Work out the finished part from the listing and answer in its coordinate system (mm). A direction names the side the tool comes from. Round coordinates to 2 decimals unless told otherwise and drop trailing zeros. Write each loop counter-clockwise with the first axis right and the second up, starting at its lowest first coordinate (ties: lowest second). Pieces come first, ordered by that corner, then holes. Notation, with made-up numbers: (-35, 53.25) - (1, 53.25) arc R24 cw to (1, 88.25) - close; hole circle Ø1 at (46.25, 12). An arc over 180 degrees is marked (long way). Write item = value, one per line. Start each with the question number.
from build123d import *

# Parameters (mm, degrees)
PAD008_DEPTH    = 4.8
SKETCH012_W     = 5
SKETCH012_H     = 110
SKETCH012_H_2   = 105
SKETCH012_W_2   = 90
SKETCH012_H_3   = 5
PAD009_DEPTH    = 0.2
PAD010_DEPTH    = 6
SKETCH024_W     = 95
SKETCH024_H     = 120
PAD021_DEPTH    = 5.67
SKETCH025_W     = 65
SKETCH025_H     = 32.5
PAD022_DEPTH    = 2
FILLET004_R     = 3.5
SKETCH029_W     = 1.25
SKETCH029_H     = 105
POCKET006_DEPTH = 5
SKETCH030_W     = 70
SKETCH030_H     = 5
POCKET007_DEPTH = 15
FILLET006_R     = 4
SKETCH032_W     = 70
SKETCH032_H     = 7.5
POCKET008_DEPTH = 4


with BuildPart() as part:
    # Sketch011 → Pad008 (new body)
    with BuildSketch(Plane.XY):
        Polygon((0, 0), (95, 0), (95, -5), (95, -110), (86.25, -110), (86.25, -5), (8.75, -5), (8.75, -110), (0, -110), (0, -5), align=None)
    extrude(amount=PAD008_DEPTH)

    # Sketch012 (on Face12 of Pad008) → Pad009 (join)
    with BuildSketch(Plane.XY.offset(4.8)):
        with Locations((2.5, -55)):
            Rectangle(SKETCH012_W, SKETCH012_H)
        with Locations((92.5, -57.5)):
            Rectangle(SKETCH012_W, SKETCH012_H_2)
        with Locations((50, -2.5)):
            Rectangle(SKETCH012_W_2, SKETCH012_H_3)
    extrude(amount=PAD009_DEPTH)

    # Pad009 Face16 → Pad010 (add)
    with BuildSketch(Plane(origin=(47.5, -40.368852, 5), x_dir=(0, 1, 0), z_dir=(0, 0, 1))):
        Polygon((40.368852, 42.5), (40.368852, 47.5), (-69.631148, 47.5), (-69.631148, 42.5), (35.368852, 42.5), (35.368852, -42.5), (-69.631148, -42.5), (-69.631148, -47.5), (35.368852, -47.5), (40.368852, -47.5), align=None)
    extrude(amount=PAD010_DEPTH)

    # Sketch024 (on Face27 of Pad010) → Pad021 (join)
    with BuildSketch(Plane.XY.offset(11)):
        with Locations((47.5, -60)):
            Rectangle(SKETCH024_W, SKETCH024_H)
        Polygon((5, -5), (90, -5), (90, -110), (82.5, -110), (82.5, -112.5), (12.5, -112.5), (12.5, -110), (5, -110), align=None, mode=Mode.SUBTRACT)
    extrude(amount=PAD021_DEPTH)

    # Sketch025 (on Face37 of Pad021) → Pad022 (join)
    with BuildSketch(Plane.XY.offset(16.67)):
        Polygon((0, -120), (95, -120), (95, -42.5), (95, -10), (95, 0), (15, 0), (0, 0), (0, -42.5), align=None)
        with Locations((47.5, -26.25)):
            Rectangle(SKETCH025_W, SKETCH025_H, mode=Mode.SUBTRACT)
    extrude(amount=PAD022_DEPTH)

    # Fillet004
    fillet004_edges = [part.edges().sort_by_distance(p)[0] for p in [
        (0, -81.25, 18.67),
        (47.5, -120, 18.67),
        (55, 0, 18.67),
        (95, -81.25, 18.67),
    ]]
    fillet(fillet004_edges, radius=FILLET004_R)

    # Sketch029 (on Face48 of Fillet004) → Pocket006 (cut)
    with BuildSketch(Plane(origin=(0, 0, 0), x_dir=(1, 0, 0), z_dir=(0, 0, -1))):
        with Locations((8.125, 57.5)):
            Rectangle(SKETCH029_W, SKETCH029_H)
        with Locations((86.875, 57.5)):
            Rectangle(SKETCH029_W, SKETCH029_H)
    extrude(amount=-POCKET006_DEPTH, mode=Mode.SUBTRACT)

    # Sketch030 (on Face48 of Pocket006) → Pocket007 (cut)
    with BuildSketch(Plane(origin=(0, 0, 0), x_dir=(1, 0, 0), z_dir=(0, 0, -1))):
        with Locations((47.5, 2.5)):
            Rectangle(SKETCH030_W, SKETCH030_H)
    extrude(amount=-POCKET007_DEPTH, mode=Mode.SUBTRACT)

    # Fillet006
    fillet006_edges = [part.edges().sort_by_distance(p)[0] for p in [
        (12.5, -2.5, 15),
        (82.5, -2.5, 15),
    ]]
    fillet(fillet006_edges, radius=FILLET006_R)

    # Sketch032 (on Face20 of Fillet006) → Pocket008 (cut)
    with BuildSketch(Plane(origin=(0, 0, 11), x_dir=(1, 0, 0), z_dir=(0, 0, -1))):
        with Locations((47.5, 116.25)):
            Rectangle(SKETCH032_W, SKETCH032_H)
    extrude(amount=-POCKET008_DEPTH, mode=Mode.SUBTRACT)


with BuildPart() as part_1:
    # Body001 placement: moved
    add(part.part.moved(Location((-15, 10, -3))))


solid = part_1.part
1. Consider line 1 (X direction, y = -76.5, z = 10.25); line 2 (X direction, y = -92, z = 1.25); line 3 (Y direction, x = -6, z = 9.25). Determine where each line is inside the solid, lowest interval first.
2. For a pull along X with two mould halves and no side action, classify faces 4 (the face through (-13.95, -50.84, 14.67)), 5 (the face through (32, -62, 15.67)), 6 (the face through (75, -47, 8)) as released by +X, released by -X, zero draft, split by the parting line, or undercut.
3. Find section D-D on y = -55. Give the vertices of the cut face in (x, z).
4. Each of these flat-tipped pins is pushed along its axis until it touches: pin 1 (0.6 mm diameter, centred on x = 38.5, z = 15, fed in from -Y); pin 2 (1.6 mm diameter, centred on x = 41, z = 14.5, fed in from +Y); pin 3 (8 mm diameter, centred on x = 76.5, z = 1, fed in from -Y). Where does it stop, or does it pass through?
5. Find section B-B on z = 4.75. Give the vertices of the cut face in (x, y), plus the area to 4 significant figures.
6. Find section C-C on y = -28. Give the vertices of the cut face in (x, z), plus the area to 3 significant figures.
7. Which of the six approach directions +Z, -Z, +X, -X, +Y, -Y give full straight-line access (tool end or side, diameter ignored) to faces 1 (the face through (-6, -100, 11)), 2 (the face through (72.5, -47, -1)), 3 (the face through (-9, -47, 1.8))?
8. Find section A-A on x = 39. Give the vertices of the cut face in (y, z), plus the area to 3 significant figures.
Answer key:
q1.line_1 = -15 to -10, 75 to 80
q1.line_2 = -15 to -7.5, 72.5 to 80
q1.line_3 = -110 to -100, 5 to 10
q2.face_4 = released by -X
q2.face_5 = zero draft
q2.face_6 = undercut
q3.outline = (-15, -3) - (-7.5, -3) - (-7.5, 1.8) - (-10, 1.8) - (-10, 13.67) - (75, 13.67) - (75, 1.8) - (72.5, 1.8) - (72.5, -3) - (80, -3) - (80, 12.17) arc R3.5 ccw to (76.5, 15.67) - (-11.5, 15.67) arc R3.5 ccw to (-15, 12.17) - close
q4.pin_1 = -108.92
q4.pin_2 = 9.65
q4.pin_3 = -100
q5.outline = (-15, -100) - (-10, -100) - (-10, 5) - (-2.5, 5) - (-2.5, 10) - (-15, 10) - close; (67.5, 5) - (75, 5) - (75, -100) - (80, -100) - (80, 10) - (67.5, 10) - close
q5.area = 1,175 mm²
q6.outline = (-15, -3) - (-7.5, -3) - (-7.5, 1.8) - (-10, 1.8) - (-10, 13.67) - (0, 13.67) - (0, 15.67) - (-11.5, 15.67) arc R3.5 ccw to (-15, 12.17) - close; (65, 13.67) - (75, 13.67) - (75, 1.8) - (72.5, 1.8) - (72.5, -3) - (80, -3) - (80, 12.17) arc R3.5 ccw to (76.5, 15.67) - (65, 15.67) - close
q6.area = 245 mm²
q7.face_1 = none
q7.face_2 = -Z, -Y
q7.face_3 = -Y
q8.outline = (-110, 12) - (-102.5, 12) - (-102.5, 13.67) - (-32.5, 13.67) - (-32.5, 15.67) - (-106.5, 15.67) arc R3.5 ccw to (-110, 12.17) - close; (0, 13.67) - (5, 13.67) - (5, 12) - (10, 12) - (10, 12.17) arc R3.5 ccw to (6.5, 15.67) - (0, 15.67) - close
q8.area = 191 mm²
